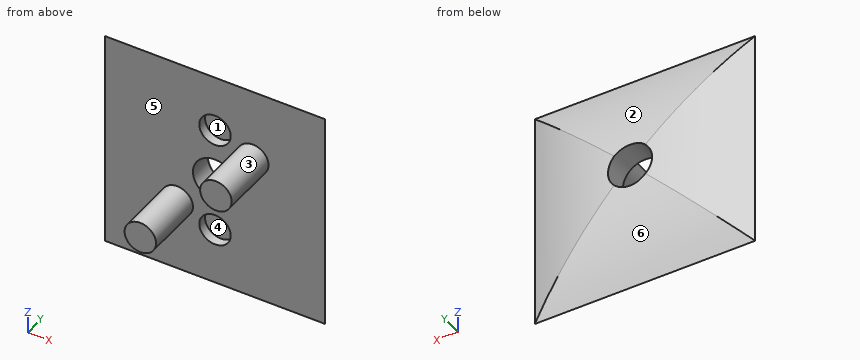
Autodesk Inventor part; units mm, degrees
ref_plane "YZ Plane" through (0, 0, 0) normal (1, 0, 0) x (0, 1, 0)
ref_plane "XZ Plane" through (0, 0, 0) normal (0, 1, 0) x (-1, 0, 0)
ref_plane "XY Plane" through (0, 0, 0) normal (0, 0, 1) x (1, 0, 0)
sketch "Sketch1" plane through (0, 0, 0) normal (0, 1, 0) x (-1, 0, 0)
  line L0 (17.5, -17.5) -> (-17.5, -17.5)
  line L1 (-17.5, -17.5) -> (-17.5, 17.5)
  line L2 (-17.5, 17.5) -> (17.5, 17.5)
  line L3 (17.5, 17.5) -> (17.5, -17.5)
  line L4 (17.5, -17.5) -> (-17.5, 17.5) construction
  line L5 (-17.5, -17.5) -> (17.5, 17.5) construction
  point P0 (0, 0)
  dimension "d0" = 35
  dimension "d1" = 35
extrude "Extrusion1" add sketch "Sketch1" along normal blind 4
sketch "Sketch3" plane through (17.5, 0, 17.5) normal (1, 0, 0) x (0, 0, -1)
  line L0 (35, 4) -> (0, 4)
  line L1 (0, 0) -> (35, 0)
  line L2 (0, 0) -> (35, 0)
  arc A0 (35, 0) -> (0, 0) centre (17.5, -36.2813) ccw
  point P0 (17.5, 4)
extrude "Extrusion3" cut sketch "Sketch3" against normal through all keep common part
sketch "Sketch4" plane through (17.5, 0, -17.5) normal (0, 0, -1) x (-1, 0, 0)
  line L0 (35, 0) -> (35, 4)
  line L1 (0, 0) -> (35, 0)
  line L2 (0, 0) -> (0, 4)
  line L3 (35, 0) -> (0, 0)
  arc A0 (35, 0) -> (0, 0) centre (17.5, -36.2812) ccw
  point P0 (17.5, 0)
  dimension "d31" = 4
extrude "Extrusion4" cut sketch "Sketch4" against normal through all keep common part
sketch "Sketch5" plane through (0, 0, 0) normal (0, -1, 0) x (1, 0, 0)
  circle A0 centre (0, 0) radius 3.5
  dimension "d14" = 7
extrude "Extrusion5" cut sketch "Sketch5" against normal through all
sketch "Sketch6" plane through (0, 0, 0) normal (0, -1, 0) x (1, 0, 0)
  circle A0 centre (-6, -6) radius 2.5
  circle A1 centre (6, 6) radius 2.5
  circle A2 centre (6, -6) radius 2.5
  circle A3 centre (-6, 6) radius 2.5
  point P0 (0, 0)
  point P1 (0, 0)
  dimension "d17" = 5
  dimension "d18" = 5
  dimension "d19" = 6
  dimension "d20" = 6
  dimension "d21" = 6
  dimension "d22" = 6
  dimension "d25" = 5
  dimension "d26" = 5
  dimension "d27" = 6
  dimension "d28" = 6
  dimension "d29" = 6
  dimension "d30" = 6
extrude "Extrusion6" add sketch "Sketch6" along normal blind 9.5 contours A0 | A1
sketch "Sketch7" plane through (0, 0, 0) normal (0, -1, 0) x (1, 0, 0)
  line L0 (-17.5, 17.5) -> (-17.5, -17.5) construction
  line L1 (-17.5, 0) -> (17.5, 0) construction
  line L2 (17.5, -17.5) -> (17.5, 17.5) construction
  circle A0 centre (0, 8.5) radius 2.5
  circle A1 centre (0, -8.5) radius 2.5
  line L3 (0, 0) -> (0, 8.5) construction
  dimension "d32" = 5
  dimension "d33" = 8.5
extrude "Extrusion7" cut sketch "Sketch7" against normal blind 1.5
equation "\"d1\" = d0"
equation "\"d17\" = d18"
equation "\"d25\" = d18"
equation "\"d26\" = d18"
properties part number "thumper-bumper-trigger-v2"
Can you work these out from the model? Positions are in its coordinate system, mm. Face numbers are marked on the shaded views. A direction names the side the tool comes from. Round coordinates to 2 decimals unless told otherwise and drop trailing zeros. Order: outer loops, then holes, each group sorted by start corner. A loop starts at its lowest first (then second) coordinate and runs counter-clockwise, first axis right, second up.
(1) If we section it at B-B (z = -1): Please give me the cut outline in (x, y).
Results are:
outline: (-17.5, 0) - (-3.35, 0) - (-3.35, 3.86) arc R40.28 ccw to start; (3.35, 0) - (17.5, 0) arc R40.28 ccw to (3.35, 3.86) - close
(2) If we section it at C-C (y = -6.75): Please give me the cut outline in (x, z).
Results are:
outline: circle Ø5 at (-6, -6); circle Ø5 at (6, 6)
(3) I'm going to push flat-ended pins straight in: pin 1 (3 mm diameter, centred on y = -3, z = 12.5, fed in from +X); pin 2 (2.5 mm diameter, centred on x = -1, z = -8, fed in from -Y); pin 3 (8 mm diameter, centred on y = -7, z = -10, fed in from -X); pin 4 (8 mm diameter, centred on x = 0.5, z = -8, fed in from -Y). Where does each tip first touch, or does it pass through?
Results are:
pin 1: passes through
pin 2: stops at y = 1.5
pin 3: stops at x = -8.5
pin 4: stops at y = 0
(4) If I drill on L1, parallel to Z at x = 0, y = 0.55; L2, parallel to Z at x = -6, y = -8.75; L3, parallel to Y at x = -6.5, z = 9.5, over which ranges is the centre line in solid material (lowest first)?
Results are:
L1: z = -16.31 to -11, -6 to -3.5, 3.5 to 6, 11 to 16.31
L2: z = -8.5 to -3.5
L3: y = 0 to 2.86
(5) We'd pull the mould along Z, two halves only. Please class the marked faces 3, 4, 5 and 6: +Z half, -Z half, draft (parallel to the pull), parting line (faces both ways), or undercut.
Results are:
face 3: parting line
face 4: undercut
face 5: draft
face 6: -Z half
(6) If we section it at A-A (x = 0): Please give me the cut outline in (y, z), plus the area to 3 significant figures.
Results are:
outline: (0, -17.5) arc R40.28 ccw to (3.85, -3.5) - (0, -3.5) - (0, -6) - (1.5, -6) - (1.5, -11) - (0, -11) - close; (0, 3.5) - (3.85, 3.5) arc R40.28 ccw to (0, 17.5) - (0, 11) - (1.5, 11) - (1.5, 6) - (0, 6) - close
area: 51.7 mm2
(7) On a 3-axis mill with a long thin cutter (end or side, diameter ignored), from which of +Z, -Z, +X, -X, +Y, -Y can I reach the whole of each face in a straight line? I mean the marked faces 1 and 2. Say none if no direction works.
Results are:
face 1: -Y
face 2: +Z, +X, -X, +Y
(8) If we section it at D-D (x = 6): Please give me the cut outline in (y, z).
Results are:
outline: (-9.5, 3.5) - (0, 3.5) - (0, -17.5) arc R40.28 ccw to (3.55, -6) - (3.55, 6) arc R40.28 ccw to (0, 17.5) - (0, 8.5) - (-9.5, 8.5) - close
